Geometry: final body of the model. Coordinates: model frame, mm. A direction names the side the tool comes from. Round coordinates to 2 decimals unless told otherwise and drop trailing zeros. Order: outer loops, then holes, each group sorted by start corner. A loop starts at its lowest first (then second) coordinate and runs counter-clockwise, first axis right, second up. Notation, with made-up numbers: (37.5, 51) -> (75.5, 51) arc R19 ccw to (75.5, 70) -> close; hole circle Ø8 at (-32.5, -9.5). An arc over 180 degrees is marked (long way). Put each result on its own line as item: value.
```python
from build123d import *

# Parameters (mm, degrees)
F0_R     = 40
F1_DEPTH = 90
F2_T     = -5
F4_R     = 5
F5_ANGLE = 180
F6_R     = 2.49999
F7_R     = 2.5


# Not quite as in the source:
# - a fillet or chamfer is up to 0.001 mm smaller than in the source, because OpenCascade refuses the exact size


with BuildPart() as f1:
    # F0 (on Top) → F1 (new body)
    with BuildSketch(Plane.XY):
        Circle(F0_R)
    extrude(amount=F1_DEPTH)

    # F2
    f2_openings = [f1.faces().sort_by_distance(p)[0] for p in [
        (0, 0, 90),
    ]]
    offset(amount=F2_T, openings=f2_openings)

    # F4 (on offset) → F5 (revolve)
    with BuildSketch(Plane.YZ.offset(37.5)):
        with Locations((0, 70)):
            Circle(F4_R)
    revolve(axis=Axis((37.5, 33.2942344248, 45), (0, 1, 0)), revolution_arc=F5_ANGLE)

    # F6 (radius 2.5 in the source; OpenCascade refuses exactly that, so slightly less here)
    f6_edges = [f1.edges().sort_by_distance(p)[0] for p in [
        (-40, 0, 90),
        (-35, 0, 90),
    ]]
    fillet(f6_edges, radius=F6_R)

    # F7
    f7_edges = [f1.edges().sort_by_distance(p)[0] for p in [
        (-40, 0, 0),
    ]]
    fillet(f7_edges, radius=F7_R)


solid = f1.part
```
1. Material intervals for probe 1 along Y at (x, z) = (0, 36); probe 2 along X at (y, z) = (3, 27); probe 3 along Y at (x, z) = (13, 37), sorted ascending.
Ans:
probe 1: -40 to -35, 35 to 40
probe 2: -39.89 to -34.87, 34.87 to 39.89, 48.32 to 60.24
probe 3: -37.83 to -32.5, 32.5 to 37.83
2. Set-up query: faces 1 (the face through (-1, 1, 0)), 2 (the face through (0, 0, 5)). Return all of +Z, -Z, +X, -X, +Y, -Y with unobstructed straight access to the full face (end or side cutting, diameter ignored); none if empty.
Ans:
face 1: -Z, +X, -X, +Y, -Y
face 2: +Z
3. Cut plane C-C on z = 83. Return loops of the section in (x, y).
Ans:
outline: circle Ø80 at (0, 0); hole circle Ø70 at (0, 0)
4. Cut plane D-D on z = 30.5. State how many separate pieces and enclosed holes the cut face has, and give its area (3 significant figures).
Ans:
separate pieces: 2
enclosed holes: 1
area: 1,280 mm²
5. Contact query for flat-ended pins moving along their axis: P1, Ø10, axis at x = 20.5, z = 41, coming from the +Y side; P2, Ø3, axis at x = -11, z = 48, coming from the +Y side; P3, Ø4, axis at x = 16, y = 0.5, coming from the +Z side. Output: stop coordinate, or through.
Ans:
P1: y = 36.87
P2: y = 38.86
P3: z = 5
